```python
from build123d import *

# Parameters (mm, degrees)
BOSS_EXTRUDE1_DEPTH     = 7
SKETCH2_W               = 44
SKETCH2_H               = 42
SKETCH2_R               = 11
BOSS_EXTRUDE3_DEPTH     = 5
BOSS_EXTRUDE4_DEPTH     = 25
CUT_EXTRUDE6_DEPTH      = 5
CUT_EXTRUDE7_DEPTH      = 63.52299577
CUT_EXTRUDE7_DEPTH_BACK = 63.52299577
SKETCH7_W               = 8
SKETCH7_H               = 12
SKETCH7_R               = 3.6
CUT_EXTRUDE9_DEPTH      = 63.522995837
CUT_EXTRUDE9_DEPTH_BACK = 2.5
SKETCH7_4_R             = 6
SKETCH7_4_R_2           = 3.6
SKETCH7_4_W             = 8
SKETCH7_4_H             = 12


with BuildPart() as part:
    # Sketch1 → Boss-Extrude1 (new body)
    with BuildSketch(Plane(origin=(0, 0, 0), x_dir=(1, 0, 0), z_dir=(0, 1, 0))):
        with BuildLine():
            Line((-29.75, 32.75), (29.75, 32.75))
            ThreePointArc((29.75, 32.75), (31.871320344, 31.871320344), (32.75, 29.75))
            Line((32.75, 29.75), (32.75, -29.75))
            ThreePointArc((32.75, -29.75), (31.871320344, -31.871320344), (29.75, -32.75))
            Line((29.75, -32.75), (-29.75, -32.75))
            ThreePointArc((-29.75, -32.75), (-31.871320344, -31.871320344), (-32.75, -29.75))
            Line((-32.75, -29.75), (-32.75, 29.75))
            ThreePointArc((-32.75, 29.75), (-31.871320344, 31.871320344), (-29.75, 32.75))
        make_face()
    extrude(amount=BOSS_EXTRUDE1_DEPTH)

    # Sketch2 → Boss-Extrude3 (add)
    with BuildSketch(Plane.XY.offset(32.75)):
        with Locations((0, 28)):
            Rectangle(SKETCH2_W, SKETCH2_H)
        with Locations((0, 26)):
            Circle(SKETCH2_R, mode=Mode.SUBTRACT)
    extrude(amount=-BOSS_EXTRUDE3_DEPTH)

    # Sketch3 → Boss-Extrude4 (add)
    with BuildSketch(Plane(origin=(0, 0, 27.75), x_dir=(-1, 0, 0), z_dir=(0, 0, -1))):
        with BuildLine():
            ThreePointArc((-3.092329219, 7), (0, 45.25), (3.092329219, 7))
            Line((3.092329219, 7), (22, 7))
            Line((22, 7), (22, 49))
            Line((22, 49), (-22, 49))
            Line((-22, 49), (-22, 7))
            Line((-22, 7), (-3.092329219, 7))
        make_face()
    extrude(amount=BOSS_EXTRUDE4_DEPTH)

    # Sketch6 → Cut-Extrude6 (cut)
    with BuildSketch(Plane.XY.offset(32.75)):
        with BuildLine():
            ThreePointArc((12.015935701, 23.616769161), (11.820419706, 22.784385288), (11.567315814, 21.967667567))
            ThreePointArc((11.567315814, 21.967667567), (12.643742012, 19.739146389), (14.87226319, 20.815572586))
            ThreePointArc((14.87226319, 20.815572586), (15.197682479, 21.865638228), (15.449060187, 22.935846064))
            ThreePointArc((15.449060187, 22.935846064), (14.072959492, 24.992869856), (12.015935701, 23.616769161))
        make_face()
        with BuildLine():
            ThreePointArc((9.966693425, 17.269162573), (9.333382629, 16.595189066), (8.654600531, 15.967034853))
            ThreePointArc((8.654600531, 15.967034853), (8.472552374, 13.498865801), (10.940721426, 13.316817644))
            ThreePointArc((10.940721426, 13.316817644), (11.798804456, 14.110899386), (12.599404896, 14.96290363))
            ThreePointArc((12.599404896, 14.96290363), (12.436178632, 17.432388837), (9.966693425, 17.269162573))
        make_face()
        with BuildLine():
            ThreePointArc((-9.275760231, 17.998576867), (-11.743929282, 18.180625024), (-11.925977439, 15.712455972))
            ThreePointArc((-11.925977439, 15.712455972), (-11.179303563, 14.905601781), (-10.378165243, 14.152798382))
            ThreePointArc((-10.378165243, 14.152798382), (-7.908680036, 14.316024645), (-8.0719063, 16.785509852))
            ThreePointArc((-8.0719063, 16.785509852), (-8.695013882, 17.371023607), (-9.275760231, 17.998576867))
        make_face()
        with BuildLine():
            ThreePointArc((-13.016102958, 23.521378654), (-15.06257598, 24.913121509), (-16.454318834, 22.866648487))
            ThreePointArc((-16.454318834, 22.866648487), (-16.195665388, 21.726485914), (-15.858108288, 20.607143472))
            ThreePointArc((-15.858108288, 20.607143472), (-13.637858233, 19.51375896), (-12.54447372, 21.734009016))
            ThreePointArc((-12.54447372, 21.734009016), (-12.811496501, 22.619459007), (-13.016102958, 23.521378654))
        make_face()
        with BuildLine():
            ThreePointArc((-2.291555584, 38.033755565), (-0.899812729, 40.080228587), (-2.946285751, 41.471971441))
            ThreePointArc((-2.946285751, 41.471971441), (-4.018378916, 41.228759992), (-5.070894944, 40.911355554))
            ThreePointArc((-5.070894944, 40.911355554), (-6.164279456, 38.691105499), (-3.944029401, 37.597720987))
            ThreePointArc((-3.944029401, 37.597720987), (-3.125405824, 37.844591105), (-2.291555584, 38.033755565))
        make_face()
        with BuildLine():
            ThreePointArc((4.361502427, 38.511586493), (6.590023605, 39.588012691), (5.513597408, 41.816533869))
            ThreePointArc((5.513597408, 41.816533869), (4.396860932, 42.1626147), (3.258703392, 42.429952897))
            ThreePointArc((3.258703392, 42.429952897), (1.201679601, 41.053852203), (2.577780295, 38.996828411))
            ThreePointArc((2.577780295, 38.996828411), (3.478113872, 38.785351927), (4.361502427, 38.511586493))
        make_face()
    extrude(amount=-CUT_EXTRUDE6_DEPTH, mode=Mode.SUBTRACT)

    # Sketch7 → Cut-Extrude7 (cut, two sides: drawn at the far end of the back side and taken through both)
    with BuildSketch(Plane(origin=(0, 7, 0), x_dir=(1, 0, 0), z_dir=(0, 1, 0)).offset(-CUT_EXTRUDE7_DEPTH_BACK)):
        with Locations((-28.75, 0)):
            Rectangle(SKETCH7_W, SKETCH7_H)
        with Locations((28.75, 0)):
            Rectangle(SKETCH7_W, SKETCH7_H)
        with Locations(Location((-20, 20, 0), (0, 0, 270))):
            Circle(SKETCH7_R)
        with Locations(Location((20, 20, 0), (0, 0, 270))):
            Circle(SKETCH7_R)
        with Locations(Location((20, -20, 0), (0, 0, 270))):
            Circle(SKETCH7_R)
        with Locations(Location((-20, -20, 0), (0, 0, 270))):
            Circle(SKETCH7_R)
    extrude(amount=CUT_EXTRUDE7_DEPTH + CUT_EXTRUDE7_DEPTH_BACK, mode=Mode.SUBTRACT)

    # Sketch7<4> → Cut-Extrude9 (cut, two sides: drawn at the far end of the back side and taken through both)
    # profile 1 of 6: a face of its own
    with BuildSketch(Plane(origin=(0, 7, 0), x_dir=(1, 0, 0), z_dir=(0, 1, 0)).offset(-CUT_EXTRUDE9_DEPTH_BACK)):
        with Locations(Location((-20, 20, 0), (0, 0, 90))):
            Circle(SKETCH7_4_R)
        with Locations(Location((-20, 20, 0), (0, 0, 270))):
            Circle(SKETCH7_4_R_2, mode=Mode.SUBTRACT)
    # profile 2 of 6: a face of its own
    with BuildSketch(Plane(origin=(0, 7, 0), x_dir=(1, 0, 0), z_dir=(0, 1, 0)).offset(-CUT_EXTRUDE9_DEPTH_BACK)):
        with Locations(Location((20, 20, 0), (0, 0, 90))):
            Circle(SKETCH7_4_R)
        with Locations(Location((20, 20, 0), (0, 0, 270))):
            Circle(SKETCH7_4_R_2, mode=Mode.SUBTRACT)
    # profile 3 of 6: a face of its own
    with BuildSketch(Plane(origin=(0, 7, 0), x_dir=(1, 0, 0), z_dir=(0, 1, 0)).offset(-CUT_EXTRUDE9_DEPTH_BACK)):
        with Locations(Location((20, -20, 0), (0, 0, 70.528779366))):
            Circle(SKETCH7_4_R)
        with Locations(Location((20, -20, 0), (0, 0, 270))):
            Circle(SKETCH7_4_R_2, mode=Mode.SUBTRACT)
    # profile 4 of 6: a face of its own
    with BuildSketch(Plane(origin=(0, 7, 0), x_dir=(1, 0, 0), z_dir=(0, 1, 0)).offset(-CUT_EXTRUDE9_DEPTH_BACK)):
        with Locations(Location((-20, -20, 0), (0, 0, 109.471220634))):
            Circle(SKETCH7_4_R)
        with Locations(Location((-20, -20, 0), (0, 0, 270))):
            Circle(SKETCH7_4_R_2, mode=Mode.SUBTRACT)
    # profile 5 of 6: a face of its own
    with BuildSketch(Plane(origin=(0, 7, 0), x_dir=(1, 0, 0), z_dir=(0, 1, 0)).offset(-CUT_EXTRUDE9_DEPTH_BACK)):
        with Locations((-28.75, 0)):
            Rectangle(SKETCH7_4_W, SKETCH7_4_H)
    # profile 6 of 6: a face of its own
    with BuildSketch(Plane(origin=(0, 7, 0), x_dir=(1, 0, 0), z_dir=(0, 1, 0)).offset(-CUT_EXTRUDE9_DEPTH_BACK)):
        with Locations((28.75, 0)):
            Rectangle(SKETCH7_4_W, SKETCH7_4_H)
    extrude(amount=CUT_EXTRUDE9_DEPTH + CUT_EXTRUDE9_DEPTH_BACK, mode=Mode.SUBTRACT)


solid = part.part
```
Work out the finished part from the listing and answer in its coordinate system (mm). A direction names the side the tool comes from. Give positions to 0.01 mm unless a question says otherwise; leave off trailing zeros. Loops run counter-clockwise (first coordinate to the right, second up) from the corner with the lowest first, then second, coordinate; pieces in that order, holes last. Notation, with made-up numbers: (40, 31.5) - (55, 31.5) arc R16 cw to (55, 60.5) - close; hole circle Ø1 at (-2.75, -2.5). An arc over 180 degrees is marked (long way). Use CSV: the item, a comma, the result in double quotes. Start each with the question number.
(1) Find section A-A, the plane x = 0. Determine the outline of the cut face in (y, z), plus the area to 3 significant figures.
(2) Find section B-B, the plane z = -20. Determine the outline of the cut face in (x, y), plus the area to 3 significant figures.
(3) A tool of negligible diameter and unlimited length cuts with its end or side. For faces 4 (the face through (22, 28, 9)), 5 (the face through (-29, 3, 6)), 6 (the face through (-16.2, 21.74, 30.28)), from which of +Z, -Z, +X, -X, +Y, -Y can it reach the whole face along a straight path? Write none if from no direction.
(4) Find the intervals of material crossed by L1, parallel to Z at x = 20, y = 5; L2, parallel to X at y = 1.25, z = -20, in increasing order.
(5) Determine the mould class of faces 1 (the face through (-13.674, 19.502, 30.285)), 2 (the face through (32.75, 3, -18)), 3 (the face through (23, 4.5, -23)) for opening direction Y: released by +Y, released by -Y, zero draft, split by the parting line, or undercut.
(6) Find section D-D, the plane y = 26. Determine the outline of the cut face in (x, z), plus the area to 3 significant figures.
(7) Each of these flat-tipped pins is pushed along its axis until it touches: pin 1 (12 mm diameter, centred on x = -17, z = -19.5, fed in from +Y); pin 2 (11.5 mm diameter, centred on x = -2, y = 31.5, fed in from -Z); pin 3 (6 mm diameter, centred on y = 29, z = 7.5, fed in from +X). Where does it stop, or does it pass through?
(8) Find section C-C, the plane z = 20. Determine the outline of the cut face in (x, y).
Results found:
1,outline,"(0, -32.75) - (7, -32.75) - (7, 27.75) - (15, 27.75) - (15, 32.75) - (0, 32.75) - close; (37, 27.75) - (45.25, 27.75) - (45.25, 2.75) - (49, 2.75) - (49, 32.75) - (37, 32.75) - close"
1,area,"652 mm^2"
2,outline,"(-32.75, 0) - (-23.6, 0) - (-23.6, 4.5) - (-26, 4.5) - (-26, 7) - (-32.75, 7) - close; (-16.4, 0) - (16.4, 0) - (16.4, 4.5) - (14, 4.5) - (14, 7) - (-14, 7) - (-14, 4.5) - (-16.4, 4.5) - close; (23.6, 0) - (32.75, 0) - (32.75, 7) - (26, 7) - (26, 4.5) - (23.6, 4.5) - close"
2,area,"334 mm^2"
3,face 4,"+Z, -Z, +X, +Y"
3,face 5,"-X, +Y, -Y"
3,face 6,"+Z, -Z"
4,L1,"-32.75 to -26, -14 to 14, 26 to 32.75"
4,L2,"-32.75 to -23.6, -16.4 to 16.4, 23.6 to 32.75"
5,face 1,"undercut"
5,face 2,"zero draft"
5,face 3,"released by +Y"
6,outline,"(-22, 2.75) - (-19.25, 2.75) - (-19.25, 14.05) arc R6 cw to (-22, 14.34) - close; (-22, 25.66) arc R6 cw to (-19.25, 25.95) - (-19.25, 27.75) - (-11, 27.75) - (-11, 32.75) - (-22, 32.75) - close; (11, 27.75) - (19.25, 27.75) - (19.25, 25.95) arc R6 cw to (22, 25.66) - (22, 32.75) - (11, 32.75) - close; (19.25, 2.75) - (22, 2.75) - (22, 14.34) arc R6 cw to (19.25, 14.05) - close"
6,area,"182 mm^2"
7,pin 1,"y = 7"
7,pin 2,"z = 27.75"
7,pin 3,"x = 22"
8,outline,"(-32.75, 0) - (-23.6, 0) - (-23.6, 4.5) - (-26, 4.5) - (-26, 7) - (-32.75, 7) - close; (-16.4, 0) - (16.4, 0) - (16.4, 4.5) - (14, 4.5) - (14, 12.79) arc R19.25 cw to (3.09, 7) - (-3.09, 7) arc R19.25 cw to (-14, 12.79) - (-14, 4.5) - (-16.4, 4.5) - close; (-14, 39.21) arc R19.25 cw to (14, 39.21) - (14, 49) - (-14, 49) - close; (23.6, 0) - (32.75, 0) - (32.75, 7) - (26, 7) - (26, 4.5) - (23.6, 4.5) - close"
